Verification items for this drawing (mm, ordinates from the low corner). Give positions to 0.01 mm unless a question says otherwise; leave off trailing zeros. Order: outer loops, then holes, each group sorted by start corner. A loop starts at its lowest first (then second) coordinate and runs counter-clockwise, first axis right, second up.
(1) Mould release check, pull along X, two halves, no side actions. Record for the marked faces 1, 2, 3 and 4: pulls with the +X half, pulls with the -X half, needs draft (parallel to the pull), parting line crosses it, or undercut.
(2) Sectioned sample at A-A on z = 9.25. Record the cut outline in (x, y).
(3) Sectioned sample at B-B on y = 43.5. Record the cut outline in (x, z) (3 decimals), plus the area to 3 significant figures.
(4) Scan lines: L1, parallel to X at y = 40, z = 5.5; L2, parallel to Y at x = 32, z = 2.75. Record each from-to range of solid material in increasing order.
(5) Gauge pin test, flat ends, axial feed: pin 1 (4 mm diameter, centred on x = 48, y = 108, fed in from +Z); pin 2 (2 mm diameter, centred on x = 14.5, z = 5, fed in from +Y); pin 3 (1.6 mm diameter, centred on x = 1, z = 4.5, fed in from +Y). Record the tip position at first contact, or that the pin passes through.
(6) Sectioned sample at C-C on x = 30. Record the cut outline in (y, z) (3 decimals), plus the area to 3 significant figures.
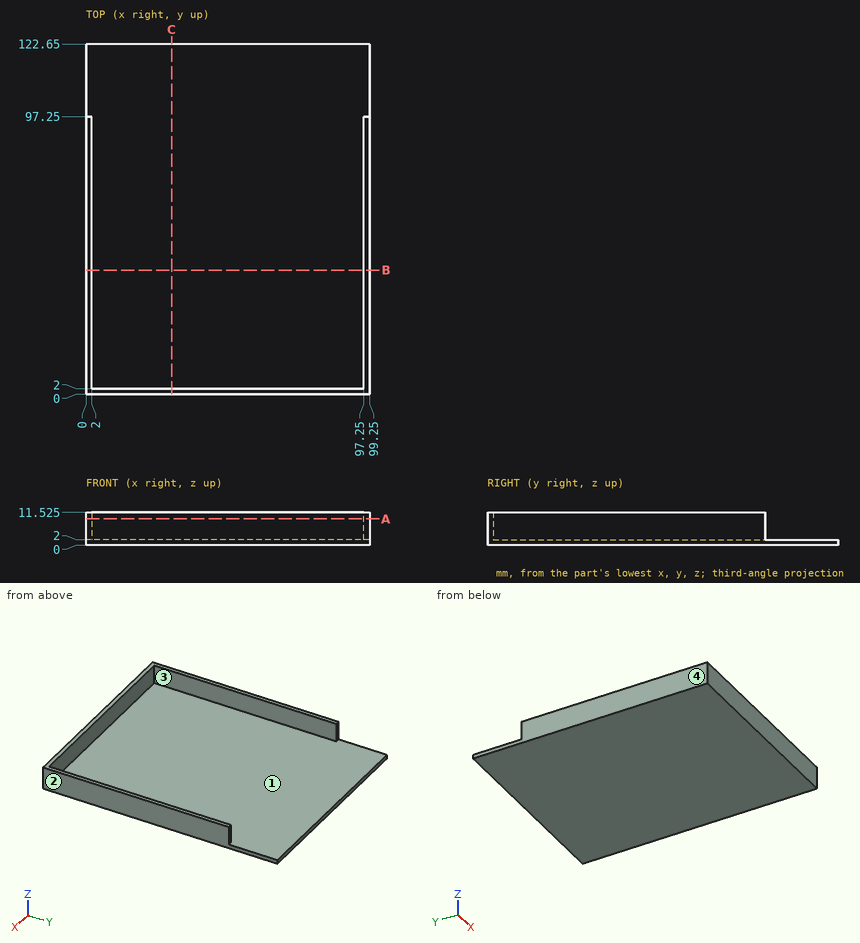
Ans:
1. face 1: undercut
1. face 2: pulls with the +X half
1. face 3: undercut
1. face 4: pulls with the -X half
2. outline: (0, 0) - (99.25, 0) - (99.25, 97.25) - (97.25, 97.25) - (97.25, 2) - (2, 2) - (2, 97.25) - (0, 97.25) - close
3. outline: (0, 0) - (99.25, 0) - (99.25, 11.525) - (97.25, 11.525) - (97.25, 2) - (2, 2) - (2, 11.525) - (0, 11.525) - close
3. area: 237 mm2
4. L1: x = 0 to 2, 97.25 to 99.25
4. L2: y = 0 to 2
5. pin 1: stops at z = 2
5. pin 2: stops at y = 2
5. pin 3: stops at y = 97.25
6. outline: (0, 0) - (122.65, 0) - (122.65, 2) - (2, 2) - (2, 11.525) - (0, 11.525) - close
6. area: 264 mm2
